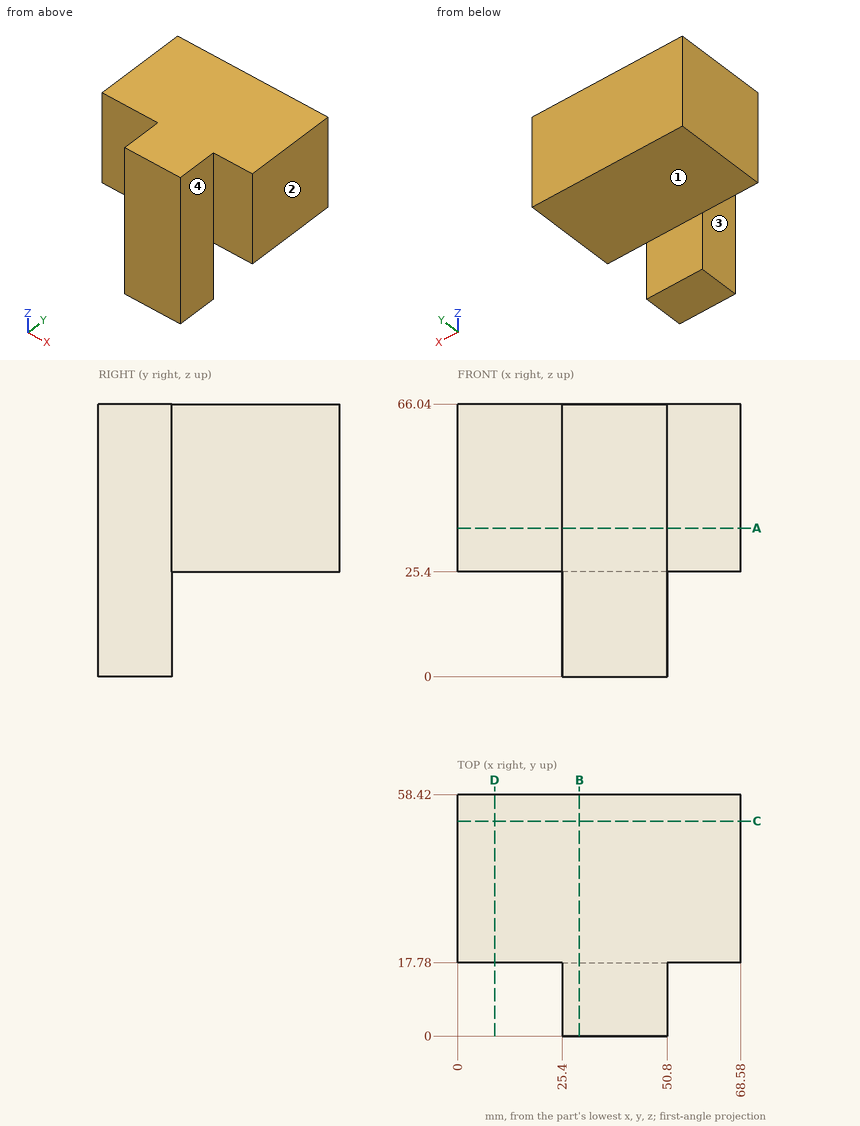
The figure shows three views and two pictorial views of one solid part (mm, origin at its lowest corner). Answer the questions. A direction names the side the tool comes from. Round coordinates to 2 decimals unless told otherwise and drop trailing zeros. Loops run counter-clockwise (first coordinate to the right, second up) from the corner with the lowest first, then second, coordinate; pieces in that order, holes last. Notation, with made-up numbers: M -19.75,-3.75 L -15.75,-3.75 A11 cw -15.75,13.25 Z; hole C -31,60 d9. An arc over 180 degrees is marked long. Write each question's results on one line, items separated by ' | '. Start each with the question number.
1) Find section C-C on y = 52. Write down the section's boundary in (x, z), plus the area to 3 significant figures.
2) Find section A-A on z = 36. Write down the section's boundary in (x, y), plus the area to 3 significant figures.
3) Find section D-D on x = 9. Write down the section's boundary in (y, z), plus the area to 3 significant figures.
4) Find section B-B on x = 29.5. Write down the section's boundary in (y, z).
5) Which of the six approach directions +Z, -Z, +X, -X, +Y, -Y give full straight-line access (tool end or side, diameter ignored) to the marked faces 1, 2, 3 and 4?
6) Each of these flat-tipped pins is pushed along its axis until it touches: pin 1 (19.5 mm diameter, centred on y = 8.5, z = 18.5, fed in from +X); pin 2 (6 mm diameter, centred on y = 12, z = 48, fed in from -X); pin 3 (12.5 mm diameter, centred on x = 17, z = 49, fed in from -Y). Where does it stop, or does it pass through?
7) Straight lines are drawn through the part: probe 1 along Z at (x, y) = (25, 50.5); probe 2 along X at (y, z) = (14, 44); probe 3 along Y at (x, z) = (34.5, 12). For each, find the intervals that lie inside material, in ascending order.
Final values:
1) outline: M 0,25.4 L 68.58,25.4 L 68.58,66.04 L 0,66.04 Z | area: 2,790 mm²
2) outline: M 0,17.78 L 25.4,17.78 L 25.4,0 L 50.8,0 L 50.8,17.78 L 68.58,17.78 L 68.58,58.42 L 0,58.42 Z | area: 3,240 mm²
3) outline: M 17.78,25.4 L 58.42,25.4 L 58.42,66.04 L 17.78,66.04 Z | area: 1,650 mm²
4) outline: M 0,0 L 17.78,0 L 17.78,25.4 L 58.42,25.4 L 58.42,66.04 L 0,66.04 Z
5) face 1: -Z, +X, -X, +Y | face 2: +Z, -Z, +X, +Y, -Y | face 3: +Z, -Z, -X, -Y | face 4: +Z, -Z, +X, -Y
6) pin 1: x = 50.8 | pin 2: x = 25.4 | pin 3: y = 17.78
7) probe 1: 25.4 to 66.04 | probe 2: 25.4 to 50.8 | probe 3: 0 to 17.78
